Part model, mm, in its own coordinate system. Face numbers are marked on the shaded views. A direction names the side the tool comes from. Coordinates: 2 decimals unless noted, no trailing zeros. Order: outer loops, then holes, each group sorted by start corner. A loop starts at its lowest first (then second) coordinate and runs counter-clockwise, first axis right, second up.
1) Pin check, flat tips, straight feed: pin 1 Ø2 at (x, z) = (-4.5, 4) entering from -Y; pin 2 Ø3 at (y, z) = (-6, 4) entering from +X; pin 3 Ø3 at (y, z) = (-14, 4) entering from -X. Stop position of each tip, or through.
2) Cut at D-D (z = 0.5). List the corners of the cut face in (x, y), and give its area (3 significant figures).
3) Cut at B-B (y = 12). List the corners of the cut face in (x, z).
4) Tool access for the marked faces 4 and 5: list every direction of +Z, -Z, +X, -X, +Y, -Y with a clear straight run to the whole face (end or side of a thin tool).
5) Mould opens along Z. For the marked faces 1, 2 and 3 say: +Z half, -Z half, draft (parallel to the pull), parting line (faces both ways), or undercut.
6) Wall check: L1, parallel to Y at x = -11.8, z = 4; L2, parallel to Z at x = -11.1, y = -14; L3, parallel to Y at x = -9.25, z = 3.25. Give the ranges that are in metal, low to high.
7) Cut at C-C (x = -17.5). List the corners of the cut face in (y, z), and give its area (3 significant figures).
8) Cut at A-A (x = -10.75). List the corners of the cut face in (y, z), and give its area (3 significant figures).
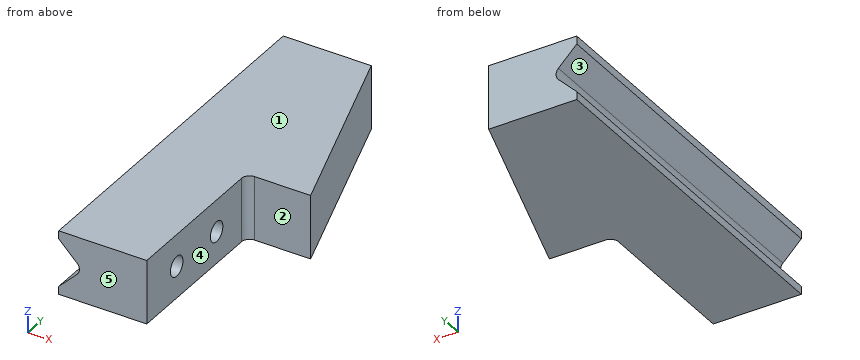
```python
from build123d import *

# Parameters (mm, degrees)
BOSS_EXTRUDE1_DEPTH       = 8
CUT_EXTRUDE1_DEPTH        = 46
M3X0_5_TAPPED_HOLE1_D     = 2.5
M3X0_5_TAPPED_HOLE1_DEPTH = 5
M3X0_5_TAPPED_HOLE1_TIP   = 0.751075774
FILLET1_R                 = 1
FILLET2_R                 = 1


with BuildPart() as part:
    # Sketch1 → Boss-Extrude1 (new body)
    with BuildSketch(Plane.XY):
        Polygon((0, 0), (-8, 0), (-8, -20), (-19, -20), (-19, 25), (-8, 25), align=None)
    extrude(amount=BOSS_EXTRUDE1_DEPTH)

    # Sketch2 → Cut-Extrude1 (cut, through all)
    with BuildSketch(Plane(origin=(0, 25, 0), x_dir=(1, 0, 0), z_dir=(0, 1, 0))):
        Polygon((-19, -4), (-19, -1), (-16, -4), (-19, -7), align=None)
    extrude(amount=-CUT_EXTRUDE1_DEPTH, mode=Mode.SUBTRACT)

    # M3x0.5 Tapped Hole1
    with Locations(Plane(origin=(-8, -6, 4), x_dir=(0, 0, 1), z_dir=(1, 0, 0))):
        with Locations((0, 0), (0, 8)):
            Hole(M3X0_5_TAPPED_HOLE1_D / 2, depth=M3X0_5_TAPPED_HOLE1_DEPTH)
            with Locations((0, 0, -(M3X0_5_TAPPED_HOLE1_DEPTH + M3X0_5_TAPPED_HOLE1_TIP / 2))):  # 118° drill point
                Cone(0, M3X0_5_TAPPED_HOLE1_D / 2, M3X0_5_TAPPED_HOLE1_TIP, mode=Mode.SUBTRACT)

    # Fillet1
    fillet1_edges = [part.edges().sort_by_distance(p)[0] for p in [
        (-16, 2.5, 4),
    ]]
    fillet(fillet1_edges, radius=FILLET1_R)

    # Fillet2
    fillet2_edges = [part.edges().sort_by_distance(p)[0] for p in [
        (-8, 0, 4),
    ]]
    fillet(fillet2_edges, radius=FILLET2_R)


solid = part.part
```
Geometry check:
1. pin 1: stops at y = 0
1. pin 2: stops at x = -8
1. pin 3: stops at x = -17.5
2. outline: (-19, -20) - (-8, -20) - (-8, -1) arc R1 cw to (-7, 0) - (0, 0) - (-8, 25) - (-19, 25) - close
2. area: 595 mm2
3. outline: (-19, 0) - (-3.84, 0) - (-3.84, 8) - (-19, 8) - (-19, 7) - (-16.71, 4.71) arc R1 cw to (-16.71, 3.29) - (-19, 1) - close
4. face 4: +Z, -Z, +X, -Y
4. face 5: +Z, -Z, +X, -X, -Y
5. face 1: +Z half
5. face 2: draft
5. face 3: undercut
6. L1: y = -20 to -15.25, -12.75 to -7.25, -4.75 to 25
6. L2: z = 0 to 2.75, 5.25 to 8
6. L3: y = -20 to -15, -13 to -7, -5 to 25
7. outline: (-20, 0) - (25, 0) - (25, 2.5) - (-20, 2.5) - close; (-20, 5.5) - (25, 5.5) - (25, 8) - (-20, 8) - close
7. area: 225 mm2
8. outline: (-20, 0) - (25, 0) - (25, 8) - (-20, 8) - close; hole circle Ø2.5 at (-14, 4); hole circle Ø2.5 at (-6, 4)
8. area: 350 mm2
